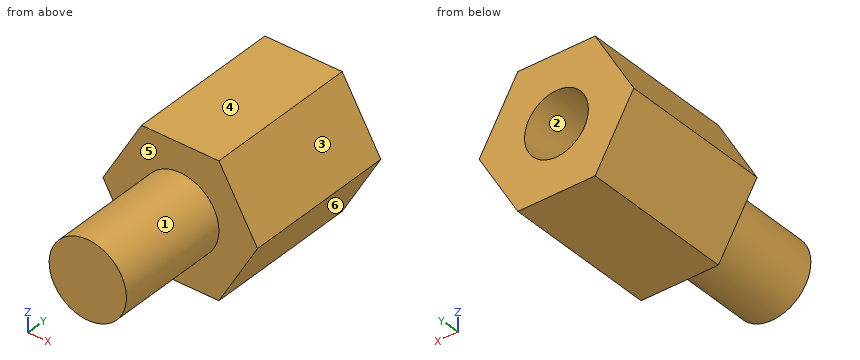
from build123d import *

# Parameters (mm, degrees)
SKETCH1_R                       = 2
BOSS_EXTRUDE1_DEPTH             = 6
BOSS_EXTRUDE2_DEPTH             = 8
TAP_DRILL_FOR_M4X0_7_TAP1_D     = 3.3
TAP_DRILL_FOR_M4X0_7_TAP1_DEPTH = 7
TAP_DRILL_FOR_M4X0_7_TAP1_TIP   = 0.991420021


with BuildPart() as part:
    # Sketch1 → Boss-Extrude1 (new body)
    with BuildSketch(Plane(origin=(0, 0, 0), x_dir=(1, 0, 0), z_dir=(0, 1, 0))):
        with Locations(Location((0, 0, 0), (0, 0, 270))):
            Circle(SKETCH1_R)
    extrude(amount=-BOSS_EXTRUDE1_DEPTH)

    # Sketch2 → Boss-Extrude2 (add)
    with BuildSketch(Plane(origin=(0, 0, 0), x_dir=(1, 0, 0), z_dir=(0, 1, 0))):
        Polygon((4, 0), (2, 3.464101615), (-2, 3.464101615), (-4, 0), (-2, -3.464101615), (2, -3.464101615), align=None)
    extrude(amount=BOSS_EXTRUDE2_DEPTH)

    # Tap Drill for M4x0.7 Tap1
    with Locations(Plane(origin=(0, 8, 0), x_dir=(1, 0, 0), z_dir=(0, 1, 0))):
        with Locations((0, 0)):
            Hole(TAP_DRILL_FOR_M4X0_7_TAP1_D / 2, depth=TAP_DRILL_FOR_M4X0_7_TAP1_DEPTH)
            with Locations((0, 0, -(TAP_DRILL_FOR_M4X0_7_TAP1_DEPTH + TAP_DRILL_FOR_M4X0_7_TAP1_TIP / 2))):  # 118° drill point
                Cone(0, TAP_DRILL_FOR_M4X0_7_TAP1_D / 2, TAP_DRILL_FOR_M4X0_7_TAP1_TIP, mode=Mode.SUBTRACT)


solid = part.part
Geometry: final body of the model. Coordinates: model frame, mm. Face numbers are marked on the shaded views. A direction names the side the tool comes from. Give positions to 0.01 mm unless a question says otherwise; leave off trailing zeros. Loops run counter-clockwise (first coordinate to the right, second up) from the corner with the lowest first, then second, coordinate; pieces in that order, holes last. Notation, with made-up numbers: (48.25, -18.5) -> (91.25, -18.5) arc R35 cw to (91.25, 13.5) -> close; hole circle Ø1 at (82, -15.5). An arc over 180 degrees is marked (long way). Put each result on its own line as item: value.
1. Pin query (flat end, axial travel): P1, Ø1.5, axis at x = 2.5, y = -3, coming from the -Z side; P2, Ø2.5, axis at x = 0, z = 0, coming from the +Y side. Return the tip coordinate at first contact, or that it passes through.
Taken from the geometry:
P1: stops at z = -0.97
P2: stops at y = 0.76
2. Cut plane C-C (z = -2.25). Return the cut outline in (x, y).
Taken from the geometry:
outline: (-2.7, 0) -> (2.7, 0) -> (2.7, 8) -> (-2.7, 8) -> close
3. Cut plane D-D (x = 2.25). Return the cut outline in (y, z), plus the area to 3 significant figures.
Taken from the geometry:
outline: (0, -3.03) -> (8, -3.03) -> (8, 3.03) -> (0, 3.03) -> close
area: 48.5 mm2
4. Cut plane B-B (y = -3). Return the cut outline in (x, z).
Taken from the geometry:
outline: circle Ø4 at (0, 0)
5. Cut plane A-A (y = 6.5). Return the cut outline in (x, z), plus the area to 3 significant figures.
Taken from the geometry:
outline: (-4, 0) -> (-2, -3.46) -> (2, -3.46) -> (4, 0) -> (2, 3.46) -> (-2, 3.46) -> close; hole circle Ø3.3 at (0, 0)
area: 33.0 mm2
6. Pull-direction query (X, two-part tool) for the marked faces 1, 2, 3 and 4; classes: released by +X, released by -X, zero draft, split by the parting line, or undercut.
Taken from the geometry:
face 1: split by the parting line
face 2: undercut
face 3: released by +X
face 4: zero draft
7. Ray query, line 1 along Z through (x, y) = (0, 6.75); line 2 along Y through (x, z) = (2, -2.5); line 3 along X through (y, z) = (-5, 0). Return the intervals inside material, ascending. Write a range as [from, to].
Taken from the geometry:
line 1: z = [-3.46, -1.65], [1.65, 3.46]
line 2: y = [0, 8]
line 3: x = [-2, 2]
8. Set-up query: the marked faces 5 and 6. Return all of +Z, -Z, +X, -X, +Y, -Y with unobstructed straight access to the full face (end or side cutting, diameter ignored); none if empty.
Taken from the geometry:
face 5: -Y
face 6: -Z, +X, +Y, -Y
